```python
from build123d import *

# Parameters (mm, degrees)
BOSS_EXTRUDE1_DEPTH     = 70
CUT_EXTRUDE1_DEPTH      = 154.378616502
CUT_EXTRUDE1_DEPTH_BACK = 154.378616502
SKETCH4_R               = 5
CUT_EXTRUDE3_DEPTH      = 161.390149323


with BuildPart() as part:
    # Sketch2 → Boss-Extrude1 (new body)
    with BuildSketch(Plane.XY):
        Polygon((0, 0), (40, 0), (40, 10), (100, 10), (100, 0), (140, 0), (140, 35), (120, 35), (120, 65), (100, 65), (100, 35), (40, 35), (40, 65), (20, 65), (20, 35), (0, 35), align=None)
    extrude(amount=-BOSS_EXTRUDE1_DEPTH)

    # Sketch3 → Cut-Extrude1 (cut, two sides: drawn at the far end of the back side and taken through both)
    with BuildSketch(Plane(origin=(120, 0, 0), x_dir=(0, 0, -1), z_dir=(1, 0, 0)).offset(-CUT_EXTRUDE1_DEPTH_BACK)):
        with BuildLine():
            Line((15, 245.293863659), (15, 65))
            ThreePointArc((15, 65), (35, 45), (55, 65))
            Line((55, 65), (55, 245.293863659))
            Line((55, 245.293863659), (55, 605.881590978))
            Line((55, 605.881590978), (15, 605.881590978))
            Line((15, 605.881590978), (15, 245.293863659))
        make_face()
    extrude(amount=CUT_EXTRUDE1_DEPTH + CUT_EXTRUDE1_DEPTH_BACK, mode=Mode.SUBTRACT)

    # Sketch4 → Cut-Extrude3 (cut, through all)
    with BuildSketch(Plane(origin=(0, 35, 0), x_dir=(1, 0, 0), z_dir=(0, 1, 0))):
        with Locations(Location((130, 35, 0), (0, 0, 180))):
            Circle(SKETCH4_R)
        with Locations(Location((10, 35, 0), (0, 0, 180))):
            Circle(SKETCH4_R)
        with Locations(Location((70, 35, 0), (0, 0, 180))):
            Circle(SKETCH4_R)
    extrude(amount=-CUT_EXTRUDE3_DEPTH, mode=Mode.SUBTRACT)


solid = part.part
```
Could you check a few things on this model? Use its own coordinates, in mm. A direction names the side the tool comes from. Round coordinates to 2 decimals unless told otherwise and drop trailing zeros. Loops run counter-clockwise (first coordinate to the right, second up) from the corner with the lowest first, then second, coordinate; pieces in that order, holes last. Notation, with made-up numbers: (13.25, 5.5) -> (49.25, 5.5) arc R18 ccw to (49.25, 9.5) -> close; hole circle Ø4 at (53, -8.75). An arc over 180 degrees is marked (long way). Put each result on its own line as item: value.
Q1. Please list where these lines run through material, in increasing order: line 1 (Z direction, x = 130, y = 34.5); line 2 (X direction, y = 47, z = -48); line 3 (Y direction, x = 83, z = -29). Write a range as from..to.
Checks:
line 1: -70..-40, -30..0
line 2: 20..40, 100..120
line 3: 10..35
Q2. I want a section at A-A on y = 4.5. Write out the boundary of the cut face in (x, z).
Checks:
outline: (0, -70) -> (40, -70) -> (40, 0) -> (0, 0) -> close; (100, -70) -> (140, -70) -> (140, 0) -> (100, 0) -> close; hole circle Ø10 at (10, -35); hole circle Ø10 at (130, -35)
Q3. Which directions (+Z, -Z, +X, -X, +Y, -Y) give clear straight access to the entire face, cutting with the end or side of a thin tool? Please do faces 1 (the flat face through (40, 5, -35)), 2 (the flat face through (120, 43, -35)), 3 (the flat face through (17, 35, -35)), 4 (the flat face through (100, 44, -35)), 5 (the flat face through (110, 65, -62)).
Checks:
face 1: +Z, -Z, -Y
face 2: +Z, -Z, +X, +Y
face 3: +Z, -Z, -X, +Y
face 4: +Z, -Z, +Y
face 5: +Z, -Z, +X, -X, +Y
Q4. I want a section at C-C on z = -35. Write out the boundary of the cut face in (x, y).
Checks:
outline: (0, 0) -> (5, 0) -> (5, 35) -> (0, 35) -> close; (15, 0) -> (40, 0) -> (40, 10) -> (65, 10) -> (65, 35) -> (40, 35) -> (40, 45) -> (20, 45) -> (20, 35) -> (15, 35) -> close; (75, 10) -> (100, 10) -> (100, 0) -> (125, 0) -> (125, 35) -> (120, 35) -> (120, 45) -> (100, 45) -> (100, 35) -> (75, 35) -> close; (135, 0) -> (140, 0) -> (140, 35) -> (135, 35) -> close
Q5. I want a section at B-B on x = 70. Write out the boundary of the cut face in (y, z).
Checks:
outline: (10, -70) -> (35, -70) -> (35, -40) -> (10, -40) -> close; (10, -30) -> (35, -30) -> (35, 0) -> (10, 0) -> close
Q6. I want a section at D-D on z = -11.5. Write out the boundary of the cut face in (x, y).
Checks:
outline: (0, 0) -> (40, 0) -> (40, 10) -> (100, 10) -> (100, 0) -> (140, 0) -> (140, 35) -> (120, 35) -> (120, 65) -> (100, 65) -> (100, 35) -> (40, 35) -> (40, 65) -> (20, 65) -> (20, 35) -> (0, 35) -> close
Q7. For pin 1 Ø10 at (x, z) = (126, -27) entering from +Y; pin 2 Ø9 at (y, z) = (51.5, -18) entering from -X; pin 3 Ø24 at (y, z) = (57.5, -30) entering from +X, each with a flat end and sliding along its axis, tell me the tip position at first contact or that it passes through.
Checks:
pin 1: y = 35
pin 2: x = 20
pin 3: x = 120
Q8. Thinking about a two-plate mould opening in X: for faces 6 (the cylindrical face through (125.381, 17.745, -36.915)), 7 (the flat face through (40, 43, -35)), 8 (the flat face through (69, 26, -70)), 9 (the flat face through (0, 18, -35)), which applies, pulls with the +X half, pulls with the -X half, needs draft (parallel to the pull), parting line crosses it, or undercut?
Checks:
face 6: undercut
face 7: undercut
face 8: needs draft
face 9: pulls with the -X half
